Input: dimensioned drawing with shaded views. Units: mm. Origin: part minimum x, y, z. Round coordinates to 2 decimals unless told otherwise and drop trailing zeros. Write each loop counter-clockwise with the first axis right and the second up, starting at its lowest first coordinate (ties: lowest second). Pieces come first, ordered by that corner, then holes. Notation, with made-up numbers: M -32,19.5 L -24,19.5 A12 ccw -24,42.5 Z; hole C 19.25,-25 d5. An arc over 180 degrees is marked long. Answer in a Markdown table with one row per item. Add a question column.
Item 1: Cut plane B-B on z = 96. Return loops of the section in (x, y) (1 decimal).
Item 2: Contact query for flat-ended pins moving along their axis: pin 1 (3 mm diameter, centred on y = 5, z = 38.5, fed in from +X); pin 2 (3 mm diameter, centred on y = 3, z = 22, fed in from -X); pin 3 (4 mm diameter, centred on x = 55.5, y = 1.5, fed in from -Z). Output: stop coordinate, or through.
Item 3: Cut plane C-C on z = 11. Return loops of the section in (x, y).
Item 4: Cut plane A-A on y = 3. Return loops of the section in (x, z), and give its area (3 significant figures).
Item 5: Cut plane D-D on z = 75. Return loops of the section in (x, y).
Item 6: Material intervals for probe 1 along X at (y, z) = (2.5, 59); probe 2 along Z at (x, y) = (86, 3.25) (1 decimal); probe 3 along Z at (x, y) = (8.5, 2.75) (1 decimal), sorted ascending.
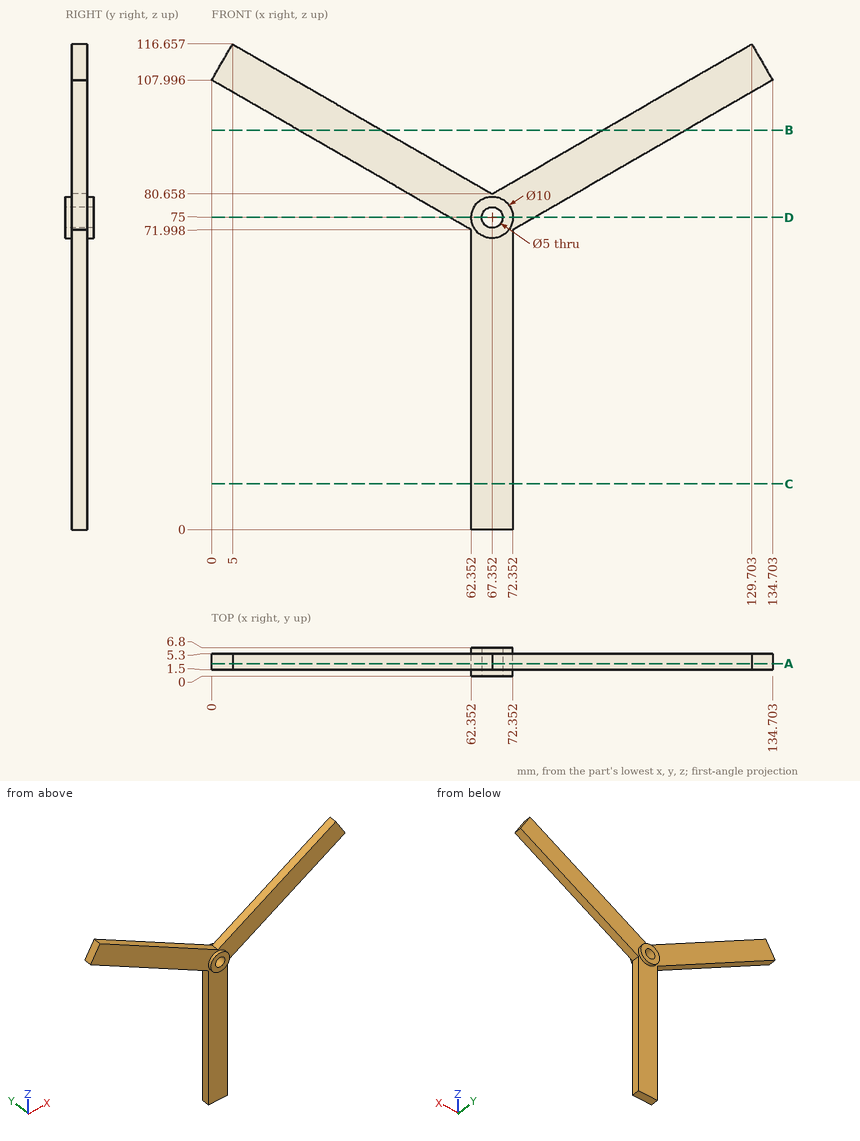
Results below:
| question | item | result |
|---|---|---|
| 1 | outline | M 20.8,1.5 L 40.8,1.5 L 40.8,5.3 L 20.8,5.3 Z; M 93.9,1.5 L 113.9,1.5 L 113.9,5.3 L 93.9,5.3 Z |
| 2 | pin 1 | x = 72.35 |
| 2 | pin 2 | x = 62.35 |
| 2 | pin 3 | z = 74.8 |
| 3 | outline | M 62.35,1.5 L 72.35,1.5 L 72.35,5.3 L 62.35,5.3 Z |
| 4 | outline | M 0,108 L 62.35,72 L 62.35,0 L 72.35,0 L 72.35,72 L 134.7,108 L 129.7,116.66 L 67.35,80.66 L 5,116.66 Z; hole C 67.35,75 d5 |
| 4 | area | 2,180 mm2 |
| 5 | outline | M 57.15,1.5 L 62.35,1.5 L 62.35,0 L 64.85,0 L 64.85,6.8 L 62.35,6.8 L 62.35,5.3 L 57.15,5.3 Z; M 69.85,0 L 72.35,0 L 72.35,1.5 L 77.55,1.5 L 77.55,5.3 L 72.35,5.3 L 72.35,6.8 L 69.85,6.8 Z |
| 6 | probe 1 | 62.35 to 72.35 |
| 6 | probe 2 | 79.9 to 91.4 |
| 6 | probe 3 | 103.1 to 114.6 |
